Here's how the part is built. I have some questions about the finished solid (model axes, mm). Face numbers are marked on the shaded views. A direction names the side the tool comes from. Coordinates: 2 decimals unless noted, no trailing zeros. Write each loop counter-clockwise with the first axis right and the second up, starting at its lowest first coordinate (ties: lowest second). Pieces come first, ordered by that corner, then holes.
from build123d import *

# Parameters (mm, degrees)
BOSS_EXTRUDE1_DEPTH = 15
SHELL1_T            = 3
SKETCH3_W           = 9
SKETCH3_H           = 11
CUT_EXTRUDE1_DEPTH  = 3
SKETCH4_R           = 2.5
CUT_EXTRUDE2_DEPTH  = 3
FILLET1_R           = 2


with BuildPart() as part:
    # Sketch1 → Boss-Extrude1 (new body)
    with BuildSketch(Plane(origin=(0, 0, 0), x_dir=(1, 0, 0), z_dir=(0, 1, 0))):
        Polygon((0, 0), (88, 0), (88, -41), (71.5, -41), (71.5, -106), (16.5, -106), (16.5, -41), (0, -41), align=None)
    extrude(amount=BOSS_EXTRUDE1_DEPTH)

    # Shell1
    shell1_openings = [part.faces().sort_by_distance(p)[0] for p in [
        (44, 15, 46.878254211),
    ]]
    offset(amount=SHELL1_T, openings=shell1_openings, kind=Kind.INTERSECTION)

    # Sketch3 → Cut-Extrude1 (cut)
    with BuildSketch(Plane(origin=(0, 0, -3), x_dir=(-1, 0, 0), z_dir=(0, 0, -1))):
        with Locations((-62, 9.5)):
            Rectangle(SKETCH3_W, SKETCH3_H)
    extrude(amount=-CUT_EXTRUDE1_DEPTH, mode=Mode.SUBTRACT)

    # Sketch4 → Cut-Extrude2 (cut)
    with BuildSketch(Plane.ZY.offset(3)):
        with Locations((31, 6)):
            Circle(SKETCH4_R)
    extrude(amount=-CUT_EXTRUDE2_DEPTH, mode=Mode.SUBTRACT)

    # Fillet1
    fillet1_edges = [part.edges().sort_by_distance(p)[0] for p in [
        (44, -3, 109),
        (13.5, -3, 76.5),
        (5.25, -3, 44),
        (-3, -3, 20.5),
        (-3, 6, -3),
        (91, 6, -3),
        (91, 6, 44),
        (74.5, 6, 44),
        (74.5, 6, 109),
        (13.5, 6, 109),
        (13.5, 6, 44),
        (-3, 6, 44),
        (44, -3, -3),
        (91, -3, 20.5),
        (82.75, -3, 44),
        (74.5, -3, 76.5),
    ]]
    fillet(fillet1_edges, radius=FILLET1_R)


solid = part.part
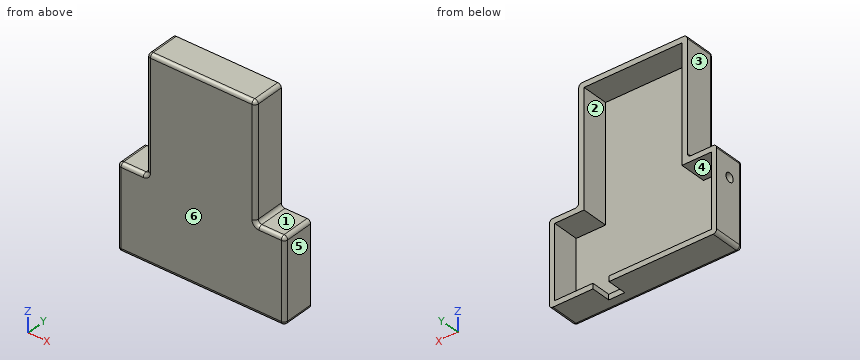
1. I want a section at D-D (z = 97). List the corners of the cut face in (x, y) for me, then the cut area to 3 significant figures.
2. On a 3-axis mill with a long thin cutter (end or side, diameter ignored), from which of +Z, -Z, +X, -X, +Y, -Y can I reach the whole of each face in a straight line? I mean the marked faces 1, 2 and 3. Say none if no direction works.
3. For pin 1 Ø1.5 at (y, z) = (9, 70.5) entering from -X; pin 2 Ø7.5 at (y, z) = (10.5, 86.5) entering from +X; pin 3 Ø1.5 at (y, z) = (9, -2) entering from +X, each with a flat end and sliding along its axis, tell me the tip position at first contact or that it passes through.
4. I want a section at A-A (z = 31). List the corners of the cut face in (x, y) for me, then the cut area to 3 significant figures.
5. Thinking about a two-plate mould opening in X: for the marked faces 4, 5 and 6, which applies, pulls with the +X half, pulls with the -X half, needs draft (parallel to the pull), parting line crosses it, or undercut?
6. I want a section at C-C (x = 32). List the corners of the cut face in (y, z) for me.
7. If I drill on line 1 (X direction, y = 7.75, z = 34); line 2 (Z direction, x = 3, y = 4.25); line 3 (Z direction, x = 26, y = 0.5), over which ranges is the centre line in solid material (lowest first)?
Response values:
1. outline: (13.5, -1) arc R2 ccw to (15.5, -3) - (72.5, -3) arc R2 ccw to (74.5, -1) - (74.5, 15) - (71.5, 15) - (71.5, 0) - (16.5, 0) - (16.5, 15) - (13.5, 15) - close
1. area: 271 mm2
2. face 1: +Z, +X, +Y, -Y
2. face 2: +Y
2. face 3: +Z, -X, +Y, -Y
3. pin 1: stops at x = 13.5
3. pin 2: stops at x = 74.5
3. pin 3: stops at x = 90.98
4. outline: (-3, -1) arc R2 ccw to (-1, -3) - (89, -3) arc R2 ccw to (91, -1) - (91, 15) - (88, 15) - (88, 0) - (0, 0) - (0, 3.5) - (-3, 3.5) - close; (-3, 8.5) - (0, 8.5) - (0, 15) - (-3, 15) - close
4. area: 355 mm2
5. face 4: undercut
5. face 5: pulls with the +X half
5. face 6: needs draft
6. outline: (-3, -1) arc R2 ccw to (-1, -3) - (15, -3) - (15, 0) - (0, 0) - (0, 106) - (15, 106) - (15, 109) - (-1, 109) arc R2 ccw to (-3, 107) - close
7. line 1: x = -3 to 0, 88 to 91
7. line 2: z = -3 to 0, 41 to 44
7. line 3: z = -3 to 0, 106 to 109
